from build123d import *

# Parameters (mm, degrees)
SKETCH_1_R          = 1.5
EXTRUDE_2_DEPTH     = 3
CUT_EXTRUDE_1_DEPTH = 10
SKETCH_4_R          = 5
CUT_EXTRUDE_2_DEPTH = 10
SKETCH_5_R          = 1.5
CUT_EXTRUDE_3_DEPTH = 10
CUT_EXTRUDE_4_DEPTH = 10


with BuildPart() as part:
    # 草图1 → 凸台-拉伸2 (new body)
    with BuildSketch(Plane(origin=(0, 0, 0), x_dir=(1, 0, 0), z_dir=(0, 1, 0))):
        with BuildLine():
            Line((-60, 70), (60, 70))
            ThreePointArc((60, 70), (130, 0), (60, -70))
            Line((60, -70), (-60, -70))
            ThreePointArc((-60, -70), (-130, 0), (-60, 70))
        make_face()
        with Locations((-122, 0)):
            Circle(SKETCH_1_R, mode=Mode.SUBTRACT)
        with Locations((122, 0)):
            Circle(SKETCH_1_R, mode=Mode.SUBTRACT)
        with Locations((-30, 60)):
            Circle(SKETCH_1_R, mode=Mode.SUBTRACT)
        with Locations((30, 60)):
            Circle(SKETCH_1_R, mode=Mode.SUBTRACT)
        with Locations((30, -60)):
            Circle(SKETCH_1_R, mode=Mode.SUBTRACT)
        with Locations((-30, -60)):
            Circle(SKETCH_1_R, mode=Mode.SUBTRACT)
    extrude(amount=EXTRUDE_2_DEPTH)

    # 草图3 → 切除-拉伸1 (cut)
    with BuildSketch(Plane(origin=(0, 3, 0), x_dir=(1, 0, 0), z_dir=(0, 1, 0))):
        with BuildLine():
            Line((-60, -70), (60, -70))
            ThreePointArc((60, -70), (130, 0), (60, 70))
            Line((60, 70), (-60, 70))
            ThreePointArc((-60, 70), (-130, 0), (-60, -70))
        make_face()
        with BuildLine():
            Line((-60, -55), (60, -55))
            ThreePointArc((60, -55), (115, 0), (60, 55))
            Line((60, 55), (-60, 55))
            ThreePointArc((-60, 55), (-115, 0), (-60, -55))
        make_face(mode=Mode.SUBTRACT)
    extrude(amount=-CUT_EXTRUDE_1_DEPTH, mode=Mode.SUBTRACT)

    # 草图4 → 切除-拉伸2 (cut)
    with BuildSketch(Plane(origin=(0, 3, 0), x_dir=(1, 0, 0), z_dir=(0, 1, 0))):
        with Locations((-60, 35)):
            Circle(SKETCH_4_R)
        with Locations((-60, -35)):
            Circle(SKETCH_4_R)
        with Locations((-80.57248383, -28.315594803)):
            Circle(SKETCH_4_R)
        with Locations((-93.28697807, -10.815594803)):
            Circle(SKETCH_4_R)
        with Locations((-93.28697807, 10.815594803)):
            Circle(SKETCH_4_R)
        with Locations((-80.57248383, 28.315594803)):
            Circle(SKETCH_4_R)
        with Locations((-40, 35)):
            Circle(SKETCH_4_R)
        with Locations((-20, 35)):
            Circle(SKETCH_4_R)
        with Locations((0, 35)):
            Circle(SKETCH_4_R)
        with Locations((20, 35)):
            Circle(SKETCH_4_R)
        with Locations((40, 35)):
            Circle(SKETCH_4_R)
        with Locations((60, 35)):
            Circle(SKETCH_4_R)
        with Locations((60, -35)):
            Circle(SKETCH_4_R)
        with Locations((40, -35)):
            Circle(SKETCH_4_R)
        with Locations((20, -35)):
            Circle(SKETCH_4_R)
        with Locations((0, -35)):
            Circle(SKETCH_4_R)
        with Locations((-20, -35)):
            Circle(SKETCH_4_R)
        with Locations((-40, -35)):
            Circle(SKETCH_4_R)
        with Locations((80.57248383, 28.315594803)):
            Circle(SKETCH_4_R)
        with Locations((93.28697807, 10.815594803)):
            Circle(SKETCH_4_R)
        with Locations((93.28697807, -10.815594803)):
            Circle(SKETCH_4_R)
        with Locations((80.57248383, -28.315594803)):
            Circle(SKETCH_4_R)
    extrude(amount=-CUT_EXTRUDE_2_DEPTH, mode=Mode.SUBTRACT)

    # 草图5 → 切除-拉伸3 (cut)
    with BuildSketch(Plane(origin=(0, 3, 0), x_dir=(1, 0, 0), z_dir=(0, 1, 0))):
        with Locations((60, 51)):
            Circle(SKETCH_5_R)
        with Locations((104.167295593, 25.5)):
            Circle(SKETCH_5_R)
        with Locations((104.167295593, -25.5)):
            Circle(SKETCH_5_R)
        with Locations((60, -51)):
            Circle(SKETCH_5_R)
        with Locations((0, -51)):
            Circle(SKETCH_5_R)
        with Locations((-60, -51)):
            Circle(SKETCH_5_R)
        with Locations((-104.167295593, -25.5)):
            Circle(SKETCH_5_R)
        with Locations((-104.167295593, 25.5)):
            Circle(SKETCH_5_R)
        with Locations((-60, 51)):
            Circle(SKETCH_5_R)
        with Locations((0, 51)):
            Circle(SKETCH_5_R)
    extrude(amount=-CUT_EXTRUDE_3_DEPTH, mode=Mode.SUBTRACT)

    # 草图6 → 切除-拉伸4 (cut)
    with BuildSketch(Plane(origin=(0, 3, 0), x_dir=(1, 0, 0), z_dir=(0, 1, 0))):
        with BuildLine():
            Line((60, 47), (-60, 47))
            ThreePointArc((-60, 47), (-107, 0), (-60, -47))
            Line((-60, -47), (60, -47))
            ThreePointArc((60, -47), (107, 0), (60, 47))
        make_face()
    extrude(amount=-CUT_EXTRUDE_4_DEPTH, mode=Mode.SUBTRACT)


solid = part.part
Check sheet for the modelled part. Datum: model origin and axes. Units: mm. A direction names the side the tool comes from. Coordinates: 2 decimals unless noted, no trailing zeros. Write each loop counter-clockwise with the first axis right and the second up, starting at its lowest first coordinate (ties: lowest second). Pieces come first, ordered by that corner, then holes.
Item 1: Cross-section at C-C on z = -43. Record the boundary of the cut face in (x, y).
Numbers:
outline: (-94.29, 0) - (-78.97, 0) - (-78.97, 3) - (-94.29, 3) - close; (78.97, 0) - (94.29, 0) - (94.29, 3) - (78.97, 3) - close
Item 2: Cross-section at A-A on y = 2.2. Count the separate pieces of the cut face and the enclosed holes in it, then the cut area to 3 significant figures.
Numbers:
separate pieces: 1
enclosed holes: 11
area: 4,410 mm2
Item 3: Mould release check, pull along X, two halves, no side actions. Record for faces 1 (the face through (106.99, 1.52, 1.03)), 2 (the face through (9, 3, 49)), 3 (the face through (114.987, 1.521, 1.209)): released by +X, released by -X, zero draft, split by the parting line, or undercut.
Numbers:
face 1: undercut
face 2: zero draft
face 3: released by +X
Item 4: Access from +Z, -Z, +X, -X, +Y, -Y to the whole of each face (thin tool, end or side, straight path). Record for faces 4 (the face through (-106.99, 1.52, -1.03)), 5 (the face through (9, 0, 49)).
Numbers:
face 4: +Y, -Y
face 5: +Z, -Z, +X, -X, -Y
Item 5: Depth check by flat-ended pin: pin 1 Ø1.5 at (y, z) = (2, 14) entering from +X. Enter the tip coordinate at first touch or a pass-through.
Numbers:
pin 1: stops at x = 113.38
Item 6: Cross-section at B-B on x = 23.5. Record the boundary of the cut face in (y, z).
Numbers:
outline: (0, -55) - (3, -55) - (3, -47) - (0, -47) - close; (0, 47) - (3, 47) - (3, 55) - (0, 55) - close
Item 7: Scan lines: probe 1 along Z at (x, y) = (0, 1.7); probe 2 along Z at (x, y) = (-53, 0.8); probe 3 along X at (y, z) = (1.55, -26.5). Record each from-to range of solid material in increasing order.
Numbers:
probe 1: z = -55 to -52.5, -49.5 to -47, 47 to 49.5, 52.5 to 55
probe 2: z = -55 to -47, 47 to 55
probe 3: x = -108.19 to -105.29, -103.05 to -98.82, 98.82 to 103.05, 105.29 to 108.19
